from build123d import *

# Parameters (mm, degrees)
F0_W     = 600
F0_H     = 200
F0_R     = 14.2
F0_R_2   = 14
F1_DEPTH = 19
F2_R     = 14.2
F2_W     = 79.5
F2_H     = 96.5
F2_R_2   = 2.75
F2_R_3   = 14
F3_DEPTH = 8.5
F4_DEPTH = 19.001
F5_R     = 5
F6_SIZE  = 3.5
F7_SIZE  = 1


# Not quite as in the source:
# - a feature names something its author has since deleted; it is built from what else it names


with BuildPart() as f1:
    # F0 (on Top) → F1 (new body)
    with BuildSketch(Plane.XY):
        Rectangle(F0_W, F0_H)
        with Locations((-125, -23.5)):
            Circle(F0_R, mode=Mode.SUBTRACT)
        with Locations((-91.5, -9.25)):
            Circle(F0_R, mode=Mode.SUBTRACT)
        with Locations((-55, -9.25)):
            Circle(F0_R, mode=Mode.SUBTRACT)
        with Locations((150, -23.5)):
            Circle(F0_R, mode=Mode.SUBTRACT)
        with Locations((183.5, -9.25)):
            Circle(F0_R, mode=Mode.SUBTRACT)
        with Locations((220, -9.25)):
            Circle(F0_R, mode=Mode.SUBTRACT)
        with Locations((-220, 5)):
            Circle(F0_R_2, mode=Mode.SUBTRACT)
        with Locations((-125, 19.25)):
            Circle(F0_R, mode=Mode.SUBTRACT)
        with Locations((-91.5, 33.5)):
            Circle(F0_R, mode=Mode.SUBTRACT)
        with Locations((-55, 33.5)):
            Circle(F0_R, mode=Mode.SUBTRACT)
        with Locations((55, 5)):
            Circle(F0_R_2, mode=Mode.SUBTRACT)
        with Locations((150, 19.25)):
            Circle(F0_R, mode=Mode.SUBTRACT)
        with Locations((183.5, 33.5)):
            Circle(F0_R, mode=Mode.SUBTRACT)
        with Locations((220, 33.5)):
            Circle(F0_R, mode=Mode.SUBTRACT)
    extrude(amount=F1_DEPTH)

    # F2 (on face) → F3 (cut)
    with BuildSketch(Plane(origin=(0, 0, 0), x_dir=(1, 0, 0), z_dir=(0, 0, -1))):
        with BuildLine():
            ThreePointArc((-98.9371975615, -50.9839381271), (-95.2950741485, -52.1171268516), (-91.5, -52.5))
            Line((-91.5, -52.5), (-55, -52.5))
            ThreePointArc((-55, -52.5), (-41.5649711575, -46.9350288425), (-36, -33.5))
            Line((-36, -33.5), (-36, 9.25))
            ThreePointArc((-36, 9.25), (-41.5649711575, 22.6850288425), (-55, 28.25))
            ThreePointArc((-55, 28.25), (-86.9227874299, 31.4657900344), (-117.5628024385, 40.9839381271))
            ThreePointArc((-117.5628024385, 40.9839381271), (-135.4807739774, 39.3478193085), (-144, 23.5))
            Line((-144, 23.5), (-144, -19.25))
            ThreePointArc((-144, -19.25), (-140.8478193085, -29.7307739774), (-132.4371975615, -36.7339381271))
            Line((-132.4371975615, -36.7339381271), (-98.9371975615, -50.9839381271))
        make_face()
        with Locations((-91.5, -33.5)):
            Circle(F2_R, mode=Mode.SUBTRACT)
        with Locations((-55, -33.5)):
            Circle(F2_R, mode=Mode.SUBTRACT)
        with Locations((-125, -19.25)):
            Circle(F2_R, mode=Mode.SUBTRACT)
        with Locations((-91.5, 9.25)):
            Circle(F2_R, mode=Mode.SUBTRACT)
        with Locations((-125, 23.5)):
            Circle(F2_R, mode=Mode.SUBTRACT)
        with Locations((-55, 9.25)):
            Circle(F2_R, mode=Mode.SUBTRACT)
        with BuildLine():
            ThreePointArc((131, -19.25), (134.1521806915, -29.7307739774), (142.5628024385, -36.7339381271))
            Line((142.5628024385, -36.7339381271), (176.0628024385, -50.9839381271))
            ThreePointArc((176.0628024385, -50.9839381271), (179.7049258515, -52.1171268516), (183.5, -52.5))
            Line((183.5, -52.5), (220, -52.5))
            ThreePointArc((220, -52.5), (233.4350288425, -46.9350288425), (239, -33.5))
            Line((239, -33.5), (239, 9.25))
            ThreePointArc((239, 9.25), (233.4350288425, 22.6850288425), (220, 28.25))
            ThreePointArc((220, 28.25), (188.0772125701, 31.4657900344), (157.4371975615, 40.9839381271))
            ThreePointArc((157.4371975615, 40.9839381271), (139.5192260226, 39.3478193085), (131, 23.5))
            Line((131, 23.5), (131, -19.25))
        make_face()
        with Locations((183.5, -33.5)):
            Circle(F2_R, mode=Mode.SUBTRACT)
        with Locations((220, -33.5)):
            Circle(F2_R, mode=Mode.SUBTRACT)
        with Locations((150, -19.25)):
            Circle(F2_R, mode=Mode.SUBTRACT)
        with Locations((183.5, 9.25)):
            Circle(F2_R, mode=Mode.SUBTRACT)
        with Locations((220, 9.25)):
            Circle(F2_R, mode=Mode.SUBTRACT)
        with Locations((150, 23.5)):
            Circle(F2_R, mode=Mode.SUBTRACT)
        with Locations((-220, -5)):
            Rectangle(F2_W, F2_H)
        with Locations((-253, -43.5)):
            Circle(F2_R_2, mode=Mode.SUBTRACT)
        with Locations((-187, -43.5)):
            Circle(F2_R_2, mode=Mode.SUBTRACT)
        with Locations((-220, -5)):
            Circle(F2_R_3, mode=Mode.SUBTRACT)
        with Locations((-253, 33.5)):
            Circle(F2_R_2, mode=Mode.SUBTRACT)
        with Locations((-187, 33.5)):
            Circle(F2_R_2, mode=Mode.SUBTRACT)
        with Locations((55, -5)):
            Rectangle(F2_W, F2_H)
        with Locations((22, -43.5)):
            Circle(F2_R_2, mode=Mode.SUBTRACT)
        with Locations((88, -43.5)):
            Circle(F2_R_2, mode=Mode.SUBTRACT)
        with Locations((55, -5)):
            Circle(F2_R_3, mode=Mode.SUBTRACT)
        with Locations((22, 33.5)):
            Circle(F2_R_2, mode=Mode.SUBTRACT)
        with Locations((88, 33.5)):
            Circle(F2_R_2, mode=Mode.SUBTRACT)
        with Locations((-253, 33.5)):
            Circle(F2_R_2)
        with Locations((-187, 33.5)):
            Circle(F2_R_2)
        with Locations((-187, -43.5)):
            Circle(F2_R_2)
        with Locations((-253, -43.5)):
            Circle(F2_R_2)
        with Locations((22, 33.5)):
            Circle(F2_R_2)
        with Locations((88, 33.5)):
            Circle(F2_R_2)
        with Locations((88, -43.5)):
            Circle(F2_R_2)
        with Locations((22, -43.5)):
            Circle(F2_R_2)
    extrude(amount=-F3_DEPTH, mode=Mode.SUBTRACT)

    # F2 (on face) → F4 (cut, through all)
    with BuildSketch(Plane(origin=(0, 0, 0), x_dir=(1, 0, 0), z_dir=(0, 0, -1))):
        with Locations((-253, 33.5)):
            Circle(F2_R_2)
        with Locations((-187, 33.5)):
            Circle(F2_R_2)
        with Locations((-187, -43.5)):
            Circle(F2_R_2)
        with Locations((-253, -43.5)):
            Circle(F2_R_2)
        with Locations((22, 33.5)):
            Circle(F2_R_2)
        with Locations((88, 33.5)):
            Circle(F2_R_2)
        with Locations((88, -43.5)):
            Circle(F2_R_2)
        with Locations((22, -43.5)):
            Circle(F2_R_2)
    extrude(amount=-F4_DEPTH, mode=Mode.SUBTRACT)

    # F5
    f5_edges = [f1.edges().sort_by_distance(p)[0] for p in [
        (-259.75, -43.25, 4.25),
        (-180.25, -43.25, 4.25),
        (-180.25, 53.25, 4.25),
        (-259.75, 53.25, 4.25),
        (15.25, 53.25, 4.25),
        (15.25, -43.25, 4.25),
        (94.75, -43.25, 4.25),
        (94.75, 53.25, 4.25),
    ]]
    fillet(f5_edges, radius=F5_R)

    # F6
    f6_edges = [f1.edges().sort_by_distance(p)[0] for p in [
        (85.25, -33.5, 19),
        (85.25, 43.5, 19),
        (19.25, 43.5, 19),
        (19.25, -33.5, 19),
        (-189.75, 43.5, 19),
        (-189.75, -33.5, 19),
        (-255.75, -33.5, 19),
        (-255.75, 43.5, 19),
    ]]
    chamfer(f6_edges, length=F6_SIZE)

    # F7
    f7_edges = [f1.edges().sort_by_distance(p)[0] for p in [
        (-234, 5, 8.5),
        (-206, 5, 13.75),
        (-234, 5, 19),
        (-139.2, 19.25, 8.5),
        (-110.8, 19.25, 13.75),
        (-139.2, 19.25, 19),
        (-105.7, 33.5, 8.5),
        (-77.3, 33.5, 13.75),
        (-105.7, 33.5, 19),
        (-139.2, -23.5, 8.5),
        (-110.8, -23.5, 13.75),
        (-139.2, -23.5, 19),
        (-105.7, -9.25, 8.5),
        (-77.3, -9.25, 13.75),
        (-105.7, -9.25, 19),
        (-69.2, -9.25, 8.5),
        (-40.8, -9.25, 13.75),
        (-69.2, -9.25, 19),
        (-69.2, 33.5, 8.5),
        (-40.8, 33.5, 13.75),
        (-69.2, 33.5, 19),
        (41, 5, 8.5),
        (69, 5, 13.75),
        (41, 5, 19),
        (135.8, 19.25, 8.5),
        (164.2, 19.25, 13.75),
        (135.8, 19.25, 19),
        (135.8, -23.5, 8.5),
        (164.2, -23.5, 13.75),
        (135.8, -23.5, 19),
        (169.3, -9.25, 8.5),
        (197.7, -9.25, 13.75),
        (169.3, -9.25, 19),
        (169.3, 33.5, 8.5),
        (197.7, 33.5, 13.75),
        (169.3, 33.5, 19),
        (205.8, 33.5, 8.5),
        (234.2, 33.5, 13.75),
        (205.8, 33.5, 19),
        (205.8, -9.25, 8.5),
        (234.2, -9.25, 13.75),
        (205.8, -9.25, 19),
        (55, 53.25, 0),
        (-220, 53.25, 0),
        (-86.922787, -31.46579, 0),
        (188.077213, -31.46579, 0),
    ]]
    chamfer(f7_edges, length=F7_SIZE)


solid = f1.part
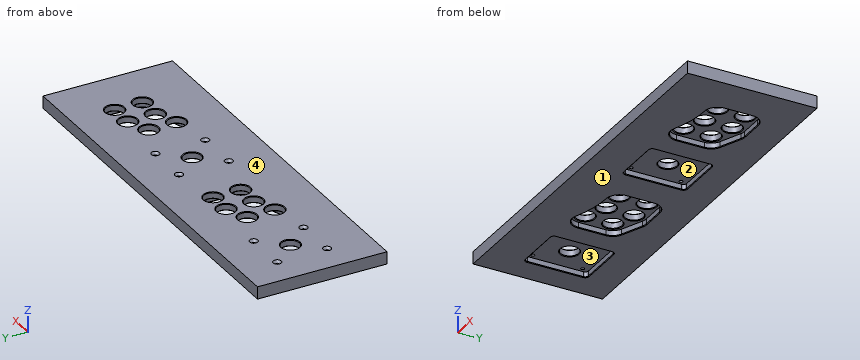
Could you check a few things on this model? Use its own coordinates, in mm. Face numbers are marked on the shaded views. A direction names the side the tool comes from. Give positions to 0.01 mm unless a question says otherwise; leave off trailing zeros. Loops run counter-clockwise (first coordinate to the right, second up) from the corner with the lowest first, then second, coordinate; pieces in that order, holes last. Notation, with made-up numbers: (14, 24) -> (56, 24) arc R20 ccw to (56, 38) -> close; hole circle Ø9 at (-4.75, 74). An arc over 180 degrees is marked (long way). Answer as CSV lines item,"result". Start each with the question number.
(1) If we section it at B-B on z = 4.5: Count the separate pieces of the cut face and the enclosed holes in it, then the cut area to 3 significant figures.
(2) Which directions (+Z, -Z, +X, -X, +Y, -Y) give clear straight access to the entire face, cutting with the end or side of a thin tool? Please do the marked faces 1 and 2.
(3) If we section it at A-A on x = 55: Write out the boundary of the cut face in (y, z).
(4) We'd pull the mould along Y, two halves only. Please class the marked faces 3 and 4: released by +Y, released by -Y, zero draft, split by the parting line, or undercut.
(5) I'm going to push a flat-ended pin straight in: pin 1 Ø7 at (x, y) = (-253, 43.5) entering from +Z. Where does the tip first touch, or does it pass through?
(6) I need wall thicknesses on probe 1 along Y at (x, z) = (183.5, 13.25); probe 2 along Y at (x, z) = (-125, 16.5); probe 3 along X at (y, z) = (5, 16). Which ranges of each line are inside material? Lowest first, please.
Computed:
1,separate pieces,"1"
1,enclosed holes,"4"
1,area,"87,500 mm2"
2,face 1,"-Z, +X, -X, +Y, -Y"
2,face 2,"-Z"
3,outline,"(-100, 0) -> (-44.25, 0) -> (-43.25, 1) -> (-43.25, 8.5) -> (-10, 8.5) -> (-9, 9.5) -> (-9, 18) -> (-10, 19) -> (-100, 19) -> close; (19, 9.5) -> (20, 8.5) -> (53.25, 8.5) -> (53.25, 1) -> (54.25, 0) -> (100, 0) -> (100, 19) -> (20, 19) -> (19, 18) -> close"
4,face 3,"undercut"
4,face 4,"zero draft"
5,pin 1,"stops at z = 16.25"
6,probe 1,"y = -100 to -23.45, 4.95 to 19.3, 47.7 to 100"
6,probe 2,"y = -100 to -37.7, -9.3 to 5.05, 33.45 to 100"
6,probe 3,"x = -300 to -234, -206 to 41, 69 to 300"
